Part model, mm, in its own coordinate system. Face numbers are marked on the shaded views. Coordinates: 2 decimals unless noted, no trailing zeros. Loops run counter-clockwise (first coordinate to the right, second up) from the corner with the lowest first, then second, coordinate; pieces in that order, holes last. Notation, with made-up numbers: M 56,58.5 L 83,58.5 A19 cw 83,89.5 Z; hole C -30.5,-10 d8. An arc over 180 degrees is marked long. Answer as a JSON object with one key per item and string values. Group by question number.
1. Saw through at C-C on x = -26. Write the cut outline in (y, z).
2. Saw through at A-A on z = 3.15. Write the cut outline in (x, y) (1 decimal).
3. Mould opens along X. For the marked faces 1, 2, 3 and 4 say: released by +X, released by -X, zero draft, split by the parting line, or undercut.
4. Saw through at B-B on y = 68. Write the cut outline in (x, z).
5. Drop flat-ended pins along their axis: pin 1 Ø1 at (x, z) = (-19.5, 3) entering from -Y; pin 2 Ø2 at (y, z) = (57.5, 0.5) entering from +X; pin 3 Ø2 at (y, z) = (66, 5) entering from -X; pin 4 Ø4.5 at (x, y) = (-21.9, 74.34) entering from +Z. Give the stop position or say it passes through.
6. Drill centre lines: L1, parallel to Y at x = 12, z = 4.1; L2, parallel to Y at x = 13.5, z = 4.7; L3, parallel to X at y = 38, z = 5.5. Where is each one in solid material? Low to high.
from build123d import *

# Parameters (mm, degrees)
ESQUISSE2_R        = 2.5
BOSS_EXTRU_1_DEPTH = 6


with BuildPart() as part:
    # Esquisse2 → Boss.-Extru.1 (new body)
    with BuildSketch(Plane.XY):
        with BuildLine():
            Line((-37.02318957, 70.208855809), (-30.229307699, 57.325290719))
            ThreePointArc((-30.229307699, 57.325290719), (-27.467524765, 54.941473247), (-23.821445078, 55.068491485))
            ThreePointArc((-23.821445078, 55.068491485), (-23.400055317, 55.248867963), (-22.977299871, 55.426019978))
            ThreePointArc((-22.977299871, 55.426019978), (-15.791425987, 55.608280441), (-10.339764744, 50.923262614))
            Line((-10.339764744, 50.923262614), (-2.578763956, 36.48608394))
            ThreePointArc((-2.578763956, 36.48608394), (0.469732203, 33.046139596), (4.735009448, 31.333260165))
            ThreePointArc((4.735009448, 31.333260165), (9.170996361, 30.332924896), (13.418131397, 28.707965042))
            ThreePointArc((13.418131397, 28.707965042), (19.90350488, 28.02390195), (25.431548669, 31.483489123))
            Line((25.431548669, 31.483489123), (30.097916289, 37.260311293))
            Line((30.097916289, 37.260311293), (37.702538192, 46.674603521))
            Line((37.702538192, 46.674603521), (49.875769926, 61.74469673))
            ThreePointArc((49.875769926, 61.74469673), (51.954878008, 69.706464375), (47.358753007, 76.532009732))
            ThreePointArc((47.358753007, 76.532009732), (8.724917717, 89.576089504), (-31.699918321, 84.232506661))
            ThreePointArc((-31.699918321, 84.232506661), (-37.526805742, 78.422186754), (-37.02318957, 70.208855809))
        make_face()
        with Locations((13.111796304, 37.260311293)):
            Circle(ESQUISSE2_R, mode=Mode.SUBTRACT)
        with Locations((-21.903504738, 74.340342212)):
            Circle(ESQUISSE2_R, mode=Mode.SUBTRACT)
    extrude(amount=BOSS_EXTRU_1_DEPTH)


solid = part.part
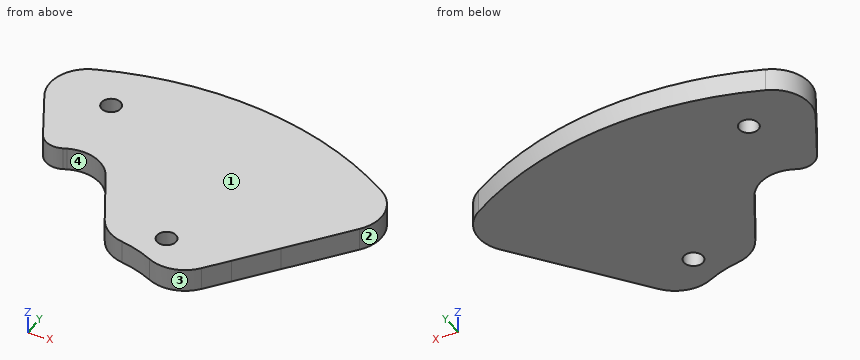
Outcome:
{
 "1": {"outline": "M 54.66,0 L 86.16,0 L 86.16,6 L 54.66,6 Z"},
 "2": {"outline": "M -37,70.2 L -30.2,57.3 A5 ccw -23.8,55.1 A60 cw -23,55.4 A10 cw -10.3,50.9 L -2.6,36.5 A10 ccw 4.7,31.3 A31.7 cw 13.4,28.7 A10 ccw 25.4,31.5 L 49.9,61.7 A10 ccw 47.4,76.5 A90 ccw -31.7,84.2 A10 ccw Z; hole C -21.9,74.3 d5; hole C 13.1,37.3 d5"},
 "3": {"face 1": "zero draft", "face 2": "released by +X", "face 3": "split by the parting line", "face 4": "undercut"},
 "4": {"outline": "M -35.86,0 L 52.1,0 L 52.1,6 L -35.86,6 Z"},
 "5": {"pin 1": "stops at y = 56.15", "pin 2": "stops at x = 47.25", "pin 3": "stops at x = -35.33", "pin 4": "passes through"},
 "6": {"L1": "y = 29.33 to 35.02, 39.5 to 89.2", "L2": "y = 28.67 to 34.79, 39.73 to 88.98", "L3": "x = -3.39 to 10.72, 15.5 to 30.7"}
}
